from build123d import *

# Parameters (mm, degrees)
SZKIC1_R                    = 9.5
DODANIE_WYCI_GNI_CIE1_DEPTH = 425
SZKIC2_R                    = 5
DODANIE_WYCI_GNI_CIE2_DEPTH = 25
SZKIC3_W                    = 3
SZKIC3_H                    = 7
DODANIE_WYCI_GNI_CIE3_DEPTH = 21
ZAOKR_GLENIE2_R             = 1.5
ZAOKR_GLENIE3_R             = 1.5


with BuildPart() as part:
    # Szkic1 → Dodanie-wyciągnięcie1 (new body)
    with BuildSketch(Plane.XY):
        Circle(SZKIC1_R)
    extrude(amount=DODANIE_WYCI_GNI_CIE1_DEPTH)

    # Szkic2 → Dodanie-wyciągnięcie2 (add)
    with BuildSketch(Plane(origin=(0, 0, 0), x_dir=(-1, 0, 0), z_dir=(0, 0, -1))):
        Circle(SZKIC2_R)
    extrude(amount=DODANIE_WYCI_GNI_CIE2_DEPTH)

    # Szkic3 → Dodanie-wyciągnięcie3 (add)
    with BuildSketch(Plane(origin=(0, 0, -2), x_dir=(-1, 0, 0), z_dir=(0, 0, -1))):
        with Locations((0, 3.5)):
            Rectangle(SZKIC3_W, SZKIC3_H)
    extrude(amount=DODANIE_WYCI_GNI_CIE3_DEPTH)

    # Zaokrąglenie2
    zaokr_glenie2_edges = [part.edges().sort_by_distance(p)[0] for p in [
        (-1.5, 5.884848004, -23),
    ]]
    fillet(zaokr_glenie2_edges, radius=ZAOKR_GLENIE2_R)

    # Zaokrąglenie3
    zaokr_glenie3_edges = [part.edges().sort_by_distance(p)[0] for p in [
        (1.5, 5.884848004, -2),
        (-1.5, 5.884848004, -2),
        (1.5, 5.884848004, -23),
    ]]
    fillet(zaokr_glenie3_edges, radius=ZAOKR_GLENIE3_R - 0.0001)  # a hair under: the kernel refuses the full size


solid = part.part
Input: part model. Units: mm. Frame: model coordinates. Give positions to 0.01 mm unless a question says otherwise; leave off trailing zeros. Order: outer loops, then holes, each group sorted by start corner. A loop starts at its lowest first (then second) coordinate and runs counter-clockwise, first axis right, second up.
Q1. Contact query for flat-ended pins moving along their axis: pin 1 Ø1.5 at (x, z) = (-6, 97) entering from -Y; pin 2 Ø0.9 at (x, z) = (-0.5, -10) entering from +Y; pin 3 Ø1.5 at (x, z) = (-3, 369) entering from +Y. Output: stop coordinate, or through.
Checked values:
pin 1: stops at y = -7.92
pin 2: stops at y = 7
pin 3: stops at y = 9.23
Q2. Ray query, probe 1 along Z at (x, y) = (-8, 3); probe 2 along Y at (x, z) = (0, 52); probe 3 along X at (y, z) = (5.75, 20). Return the intervals inside material, ascending.
Checked values:
probe 1: z = 0 to 425
probe 2: y = -9.5 to 9.5
probe 3: x = -7.56 to 7.56
Q3. Section A-A on y = 0. Output: boundary loops of the cut face in (x, z).
Checked values:
outline: (-9.5, 0) - (-5, 0) - (-5, -25) - (5, -25) - (5, 0) - (9.5, 0) - (9.5, 425) - (-9.5, 425) - close
Q4. Section B-B on z = 328. Output: boundary loops of the cut face in (x, y).
Checked values:
outline: circle Ø19 at (0, 0)
